Build history of the part. All positions in model axes, mm. Face numbers are marked on the shaded views. A direction names the side the tool comes from. Coordinates: 2 decimals unless noted, no trailing zeros. Write each loop counter-clockwise with the first axis right and the second up, starting at its lowest first coordinate (ties: lowest second). Pieces come first, ordered by that corner, then holes. Notation, with made-up numbers: M -9,-15.75 L 40,-15.75 A25 ccw 40,15.25 Z; hole C -35.75,49.25 d4. An arc over 180 degrees is marked long. Use CSV: the item, a comma, the result in double quotes. Start each with the question number.
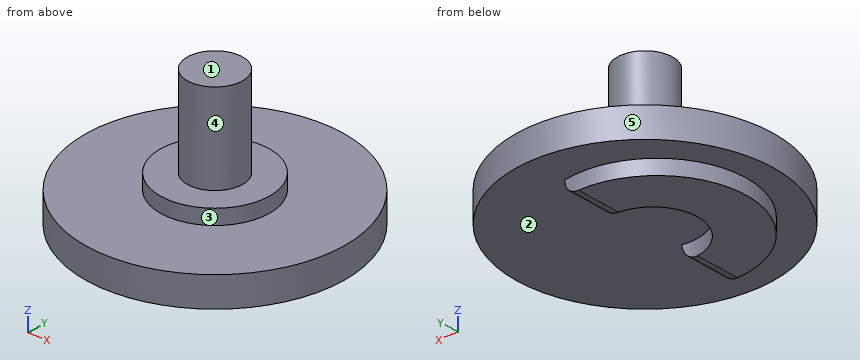
```python
from build123d import *

# Parameters (mm, degrees)
F0_R     = 2.35
F1_DEPTH = 11.43
F0_R_2   = 4.636
F2_DEPTH = 3.81
F0_R_3   = 11
F3_DEPTH = 2.54
F5_DEPTH = 1.27
F6_R     = 1.26999


# Not quite as in the source:
# - a fillet or chamfer is up to 0.001 mm smaller than in the source, because OpenCascade refuses the exact size


with BuildPart() as f1:
    # F0 (on Top) → F1 (new body)
    with BuildSketch(Plane.XY):
        Circle(F0_R)
    extrude(amount=F1_DEPTH)

    # F0 (on Top) → F2 (join)
    with BuildSketch(Plane.XY):
        Circle(F0_R_2)
        Circle(F0_R, mode=Mode.SUBTRACT)
    extrude(amount=F2_DEPTH)

    # F0 (on Top) → F3 (join)
    with BuildSketch(Plane.XY):
        Circle(F0_R_3)
        Circle(F0_R_2, mode=Mode.SUBTRACT)
    extrude(amount=F3_DEPTH)

    # F4 (on face) → F5 (join)
    with BuildSketch(Plane.XY):
        with BuildLine():
            Line((0, 3.888), (0, 7.698))
            ThreePointArc((0, 7.698), (-8.8259203096, 0.174027897), (0, -7.349944206))
            Line((0, -7.349944206), (0, -3.5482488357))
            ThreePointArc((0, -3.5482488357), (-4.6416554656, 0.1698755822), (0, 3.888))
        make_face()
    extrude(amount=-F5_DEPTH)

    # F6 (radius 1.27 in the source; OpenCascade refuses exactly that, so slightly less here)
    f6_edges = [f1.edges().sort_by_distance(p)[0] for p in [
        (0, 5.793, -1.27),
        (0, -5.449097, -1.27),
    ]]
    fillet(f6_edges, radius=F6_R)


solid = f1.part
```
1. Slice it at D-D (y = 1.25). List the corners of the cut face in (x, z), and give its area (3 significant figures).
2. Flat gauge pins, fed straight in: pin 1 (4 mm diameter, centred on y = 6, z = 5.5, fed in from -X) (3 decimals); pin 2 (4 mm diameter, centred on x = -5, y = -5.5, fed in from +Z); pin 3 (2 mm diameter, centred on x = -7.5, y = 7.5, fed in from -Z). Where does each tip first touch, or does it go through?
3. Drill centre lines: line 1 along Z through (x, y) = (2, 8.25); line 2 along X through (y, z) = (0, -0.5); line 3 along Z through (x, y) = (-2, -2). Where is each one in solid material? Low to high. Write a range as from..to.
4. Pull direction Z, two halves, no side cores. Call the marked faces 1, 2 and 3: pulls with the +Z half, pulls with the -Z half, needs draft (parallel to the pull), parting line crosses it, or undercut.
5. Slice it at C-C (z = 5). List the corners of the cut face in (x, y), and give its area (3 significant figures).
6. Slice it at A-A (x = 4). List the corners of the cut face in (y, z), and give its area (3 significant figures).
7. 3-axis set-ups, long thin cutter, end or side, ignore diameter. For the marked faces 4 and 5: which of +Z, -Z, +X, -X, +Y, -Y reach the whole face in a straight line?
Established:
1,outline,"M -10.93,0 L -8.75,0 L -8.75,-1.27 L -4.49,-1.27 L -4.49,0 L 10.93,0 L 10.93,2.54 L 4.46,2.54 L 4.46,3.81 L 1.99,3.81 L 1.99,11.43 L -1.99,11.43 L -1.99,3.81 L -4.46,3.81 L -4.46,2.54 L -10.93,2.54 Z"
1,area,"103 mm2"
2,pin 1,"passes through"
2,pin 2,"stops at z = 2.54"
2,pin 3,"stops at z = 0"
3,line 1,"z = 0..2.54"
3,line 2,"x = -8.82..-4.64"
3,line 3,"z = 0..3.81"
4,face 1,"pulls with the +Z half"
4,face 2,"pulls with the -Z half"
4,face 3,"needs draft"
5,outline,"C 0,0 d4.7"
5,area,"17.3 mm2"
6,outline,"M -10.25,0 L 10.25,0 L 10.25,2.54 L 2.34,2.54 L 2.34,3.81 L -2.34,3.81 L -2.34,2.54 L -10.25,2.54 Z"
6,area,"58.0 mm2"
7,face 4,"+Z"
7,face 5,"+Z, -Z"
